Autodesk Inventor part; units mm, degrees
ref_plane "YZ Plane" through (0, 0, 0) normal (1, 0, 0) x (0, 1, 0)
ref_plane "XZ Plane" through (0, 0, 0) normal (0, 1, 0) x (-1, 0, 0)
ref_plane "XY Plane" through (0, 0, 0) normal (0, 0, 1) x (1, 0, 0)
sketch "Szkic1" plane through (0, 0, 0) normal (0, 1, 0) x (-1, 0, 0)
  line L0 (0, 0) -> (37, 0)
  line L1 (37, 0) -> (37, -3)
  line L2 (37, -3) -> (0, -3)
  line L3 (0, -3) -> (0, 0)
  line L4 (37, 0) -> (34, 0)
  line L5 (34, 0) -> (34, -60)
  line L6 (34, -60) -> (37, -60)
  line L7 (37, -60) -> (37, 0)
  line L8 (37, -60) -> (0, -60)
  line L9 (0, -60) -> (0, -57)
  line L10 (0, -57) -> (37, -57)
  line L11 (37, -57) -> (37, -60)
  point P0 (34, -3)
  point P1 (34, -57)
  dimension "d0" = 37
  dimension "d1" = 3
  dimension "d2" = 3
  dimension "d3" = 60
  dimension "d4" = 37
  dimension "d5" = 3
extrude "Wyciągnięcie proste1" add sketch "Szkic1" along normal blind 8
sketch "Szkic2" plane through (-37, 0, 0) normal (0, 0, 1) x (1, 0, 0)
  circle A0 centre (9, 3) radius 1.95
  line L0 (0, 0) -> (37, 0)
  line L1 (0, 0) -> (0, 8)
  circle A1 centre (4.5, 3) radius 0.85
  circle A2 centre (13.5, 3) radius 0.85
  circle A3 centre (18.5, 3) radius 0.85
  circle A4 centre (27.5, 3) radius 0.85
  circle A5 centre (23, 3) radius 1.95
  dimension "d8" = 3.9
  dimension "d9" = 3
  dimension "d10" = 9
  dimension "d11" = 1.7
  dimension "d12" = 1.7
  dimension "d13" = 1.7
  dimension "d14" = 1.7
  dimension "d15" = 4.5
  dimension "d16" = 3
  dimension "d17" = 13.5
  dimension "d18" = 3
  dimension "d19" = 5
  dimension "d20" = 3
  dimension "d21" = 3.9
  dimension "d22" = 4.5
  dimension "d23" = 3
  dimension "d24" = 4.5
  dimension "d25" = 3
sketch "Szkic3" plane through (0, 0, -60) normal (0, 0, -1) x (-1, 0, 0)
  circle A0 centre (28, 3) radius 1.95
  circle A1 centre (32.5, 3) radius 0.85
  circle A2 centre (23.5, 3) radius 0.85
  circle A3 centre (18.5, 3) radius 0.85
  circle A4 centre (14, 3) radius 1.95
  circle A5 centre (9.5, 3) radius 0.85
  point P0 (0, 0)
extrude "Wyciągnięcie proste2" cut sketch "Szkic3" against normal blind 3
extrude "Wyciągnięcie proste3" cut sketch "Szkic2" against normal blind 3
sketch "Szkic4" plane through (0, 8, 0) normal (0, 1, 0) x (1, 0, 0)
  line L0 (0, 0) -> (0, 3)
  line L1 (0, 0) -> (-6, 0)
  line L2 (-6, 0) -> (-6, 6)
  line L3 (-6, 6) -> (0, 6)
  line L4 (0, 6) -> (0, 0)
  line L5 (0, 60) -> (-37, 60)
  line L6 (0, 60) -> (-6, 60)
  line L7 (-6, 60) -> (-6, 54)
  line L8 (-6, 54) -> (0, 54)
  line L9 (0, 54) -> (0, 60)
  dimension "d30" = 6
  dimension "d31" = 6
  dimension "d32" = 6
  dimension "d33" = 6
extrude "Wyciągnięcie proste4" add sketch "Szkic4" against normal blind 8
sketch "Szkic5" plane through (0, 0, 0) normal (0, -1, 0) x (1, 0, 0)
  line L0 (-6, -6) -> (0, -6)
  line L1 (0, -6) -> (-6, -6)
  line L2 (-6, -6) -> (-6, 0)
  line L3 (-6, 0) -> (0, 0)
  line L4 (0, 0) -> (0, -6)
  line L5 (0, -54) -> (-6, -54)
  line L6 (0, -60) -> (-37, -60)
  line L7 (0, -54) -> (-6, -54)
  line L8 (-6, -54) -> (-6, -60)
  line L9 (-6, -60) -> (0, -60)
  line L10 (0, -60) -> (0, -54)
extrude "Wyciągnięcie proste5" cut sketch "Szkic5" against normal blind 3
sketch "Szkic6" plane through (0, 3, 0) normal (0, -1, 0) x (1, 0, 0)
  circle A0 centre (-3, -3) radius 2
  circle A1 centre (-3, -57) radius 2
  line L0 (0, 0) -> (0, -6)
  line L1 (-6, 0) -> (0, 0)
  line L2 (-6, -54) -> (0, -54)
  line L3 (0, -54) -> (0, -60)
  point P0 (-3, -54)
  dimension "d38" = 4
  dimension "d39" = 4
  dimension "d40" = 3
  dimension "d41" = 3
  dimension "d42" = 3
  dimension "d43" = 3
extrude "Wyciągnięcie proste6" cut sketch "Szkic6" against normal blind 4
sketch "Szkic7" plane through (-34, 0, -3) normal (0, 0, -1) x (-1, 0, 0)
  circle A0 centre (-6, 3) radius 1.95
  circle A1 centre (-6, 3) radius 2.2
  circle A2 centre (-20, 3) radius 1.95
  circle A3 centre (-20, 3) radius 2.2
  point P0 (-34, 0)
  dimension "d46" = 4.4
  dimension "d47" = 4.4
extrude "Wyciągnięcie proste7" cut sketch "Szkic7" against normal blind 0.6 contours A0 | A1 | A2 | A3
sketch "Szkic8" plane through (-34, 0, -57) normal (0, 0, 1) x (1, 0, 0)
  circle A0 centre (20, 3) radius 2.2
  circle A1 centre (20, 3) radius 2.2
  circle A2 centre (6, 3) radius 2.2
  circle A3 centre (6, 3) radius 2.2
  point P0 (34, 0)
  dimension "d50" = 4.4
  dimension "d51" = 4.4
extrude "Wyciągnięcie proste8" cut sketch "Szkic8" against normal blind 0.6
fillet "Fillet1" radius 3 4 edges at (0, 5.5, 0) (0, 5.5, -6) (0, 5.5, -54) (0, 5.5, -60)
fillet "Zaokrąglenie2" radius 3 2 edges at (-6, 5.5, -54) (-6, 5.5, -6)
properties part number "bmw" material "Tworzywo sztuczne PET"
Can you work these out from the model? Positions are in its coordinate system, mm. A direction names the side the tool comes from. Coordinates: 2 decimals unless noted, no trailing zeros. Order: outer loops, then holes, each group sorted by start corner. A loop starts at its lowest first (then second) coordinate and runs counter-clockwise, first axis right, second up.
1. If we section it at A-A (x = -18.5): Please give me the cut outline in (y, z).
2. For faces 1 (the face through (-6, 1, -2)), 2 (the face through (-3, 5, -5)), 3 (the face through (-9.892, 2.246, -58.521)), 4 (the face through (-16.1, 3.66, -2.7)), 5 (the face through (-20, 4, -3)), which set-ups out of +Z, -Z, +X, -X, +Y, -Y let a thin tool reach every point of the face, with its end or its side?
3. Thinking about a two-plate mould opening in Y: for faces 6 (the face through (-25.802, 3.097, -2.704)), 7 (the face through (-3, 7, -57)), 8 (the face through (-0.9, 5.46, -5.14)), which applies, +Y half, -Y half, draft (parallel to the pull), parting line (faces both ways), or undercut?
4. If we section it at B-B (y = 6): Give the number of separate pieces and of enclosed holes in the cut face, then the cut area to 3 significant figures.
5. If we section it at C-C (z = -29.5): Please give me the cut outline in (x, y).
6. I'm going to push flat-ended pins straight in: pin 1 (2.5 mm diameter, centred on x = -14, y = 3, fed in from +Z); pin 2 (1.5 mm diameter, centred on y = 1.5, z = -1.5, fed in from +X). Where does each tip first touch, or does it pass through?
7. I need wall thicknesses on line 1 (Y direction, x = -32.5, z = -58.45); line 2 (Z direction, x = -24, y = 6.5); line 3 (Y direction, x = -14, z = -57.45). Which ranges of each line are inside material? Lowest first, please.
Entries:
1. outline: (0, -60) - (2.15, -60) - (2.15, -57) - (0, -57) - close; (0, -3) - (2.15, -3) - (2.15, 0) - (0, 0) - close; (3.85, -60) - (8, -60) - (8, -57) - (3.85, -57) - close; (3.85, -3) - (8, -3) - (8, 0) - (3.85, 0) - close
2. face 1: +Z, -Z, +X, -Y
2. face 2: -Y
2. face 3: +Z, -Z
2. face 4: none
2. face 5: +Y, -Y
3. face 6: undercut
3. face 7: -Y half
3. face 8: draft
4. separate pieces: 1
4. enclosed holes: 2
4. area: 383 mm2
5. outline: (-37, 0) - (-34, 0) - (-34, 8) - (-37, 8) - close
6. pin 1: passes through
6. pin 2: stops at x = -6
7. line 1: y = 0 to 2.15, 3.85 to 8
7. line 2: z = -60 to -57, -3 to 0
7. line 3: y = 0 to 0.8, 5.2 to 8
